Geometry: final body of the model. Coordinates: model frame, mm. A direction names the side the tool comes from. Coordinates: 2 decimals unless noted, no trailing zeros. Write each loop counter-clockwise with the first axis right and the second up, starting at its lowest first coordinate (ties: lowest second). Pieces come first, ordered by that corner, then holes. Notation, with made-up numbers: (20, 9.25) - (54, 9.25) arc R27 ccw to (54, 43.25) - close; hole circle Ø6 at (62.5, 9.25). An arc over 180 degrees is marked (long way). Answer as a JSON object with one key per item and string values. Group by question number.
Item 1: Set-up query: faces 5 (the cylindrical face through (11.923, -3.755, -33.951)), 6 (the cylindrical face through (11.446, -3.604, -20.867)), 7 (the flat face through (0, 0, 3.5)). Return all of +Z, -Z, +X, -X, +Y, -Y with unobstructed straight access to the full face (end or side cutting, diameter ignored); none if empty.
Item 2: First-contact query: pin 1 Ø2 at (y, z) = (-7, -25) entering from +X; pin 2 Ø12 at (x, z) = (10.5, -30) entering from +Y; pin 3 Ø3 at (x, z) = (-2.5, -25.5) entering from +Y. Flat tips, straight axial feed; report the tip coordinate or a pass-through.
Item 3: Mould query, pull axis Z, two halves, no side actions, for faces 1 (the flat face through (-6.05, 11.14, -38.5)), 2 (the flat face through (6.05, 11.14, -37.5)), 3 (the cylindrical face through (6.34, 12.2, -41.49)), 4 (the flat face through (-7, -10, -30.5)). Classes: pulls with the +Z half, pulls with the -Z half, needs draft (parallel to the pull), parting line crosses it, or undercut.
Item 4: Line query: line 1 along Z through (x, y) = (9.5, 9.25); line 2 along X through (y, z) = (-0.5, -27.5); line 3 along X through (y, z) = (4.25, -26). Output: solid intervals per line, ascending. Write a range as from..to.
Item 5: Section D-D on z = -24.5. Return loops of the section in (x, y), and give its area (3 significant figures).
Item 6: Section C-C on z = -9.5. Return loops of the section in (x, y).
Item 7: Section A-A on y = 0. Return loops of the section in (x, z), and give its area (3 significant figures).
```python
from build123d import *

# Parameters (mm, degrees)
SKETCH1_R           = 12.5
BOSS_EXTRUDE1_DEPTH = 3.5
SKETCH5_R           = 9.75
CUT_EXTRUDE2_DEPTH  = 5
CUT_EXTRUDE2_DRAFT  = -45


with BuildPart() as part:
    # Sketch1 → Boss-Extrude1 (new, symmetric)
    with BuildSketch(Plane.XY):
        Circle(SKETCH1_R)
    extrude(amount=BOSS_EXTRUDE1_DEPTH, both=True)

    # Sketch4 → Revolve1 (revolve)
    with BuildSketch(Plane(origin=(0, 0, 0), x_dir=(1, 0, 0), z_dir=(0, 1, 0)), mode=Mode.PRIVATE) as revolve1_sk:
        Polygon((-12.5, 3.5), (0, 3.5), (0, 42.5), (-13.75, 42.5), (-13.75, 40.5), (-12.5, 40.5), (-12.5, 38.5), (-13.75, 38.5), (-13.75, 37.5), (-12.5, 37.5), (-12.5, 30.5), (-12, 30.5), (-12, 11.5), (-12.5, 11.5), align=None)
    revolve(revolve1_sk.sketch.rotate(Axis((0, 0, -3.5), (0, 0, -1)), 180), axis=Axis((0, 0, -3.5), (0, 0, -1)))


with BuildPart() as cut_extrude2_tool:
    # Sketch5 → Cut-Extrude2 (with draft: the straight prism first)
    with BuildSketch(Plane(origin=(0, 0, -42.5), x_dir=(-1, 0, 0), z_dir=(0, 0, -1))):
        Circle(SKETCH5_R)
    extrude(amount=-CUT_EXTRUDE2_DEPTH)
    # Cut-Extrude2: the draft: its side faces are tilted about the plane it starts from
    cut_extrude2_sides = [cut_extrude2_tool.faces().sort_by_distance(p)[0] for p in [
        (9.75, 0, -40),
    ]]
    draft(cut_extrude2_sides, Plane(origin=(0, 0, -42.5), x_dir=(-1, 0, 0), z_dir=(0, 0, -1)), CUT_EXTRUDE2_DRAFT)


with BuildPart() as part_1:
    add(part.part)

    # Cut-Extrude2: cut by cut_extrude2_tool
    add(cut_extrude2_tool.part, mode=Mode.SUBTRACT)

    # Sketch6 → Revolve2 (revolve)
    with BuildSketch(Plane(origin=(0, 0, 0), x_dir=(1, 0, 0), z_dir=(0, 1, 0))):
        with BuildLine():
            Line((-4.75, 37.5), (0, 37.5))
            Line((0, 37.5), (0, 42.25))
            ThreePointArc((0, 42.25), (-3.358757211, 40.858757211), (-4.75, 37.5))
        make_face()
    revolve(axis=Axis((0, 0, -37.5), (0, 0, -1)))


solid = part_1.part
```
Checks:
{
 "1": {"face 5": "+Z", "face 6": "none", "face 7": "+Z, +X, -X, +Y, -Y"},
 "2": {"pin 1": "x = 10.39", "pin 2": "y = 11.65", "pin 3": "y = 11.96"},
 "3": {"face 1": "undercut", "face 2": "pulls with the +Z half", "face 3": "needs draft", "face 4": "undercut"},
 "4": {"line 1": "-42.5..-40.5, -38.5..-37.5", "line 2": "-11.99..11.99", "line 3": "-11.22..11.22"},
 "5": {"outline": "circle Ø24 at (0, 0)", "area": "452 mm^2"},
 "6": {"outline": "circle Ø25 at (0, 0)"},
 "7": {"outline": "(-13.75, -42.5) - (-9.75, -42.5) - (-4.75, -37.5) arc R4.75 ccw to (4.75, -37.5) - (9.75, -42.5) - (13.75, -42.5) - (13.75, -40.5) - (12.5, -40.5) - (12.5, -38.5) - (13.75, -38.5) - (13.75, -37.5) - (12.5, -37.5) - (12.5, -30.5) - (12, -30.5) - (12, -11.5) - (12.5, -11.5) - (12.5, 3.5) - (-12.5, 3.5) - (-12.5, -11.5) - (-12, -11.5) - (-12, -30.5) - (-12.5, -30.5) - (-12.5, -37.5) - (-13.75, -37.5) - (-13.75, -38.5) - (-12.5, -38.5) - (-12.5, -40.5) - (-13.75, -40.5) - close", "area": "1,100 mm^2"}
}
